Input: part model. Units: mm. Frame: model coordinates. A direction names the side the tool comes from. Round coordinates to 2 decimals unless told otherwise and drop trailing zeros. Order: outer loops, then holes, each group sorted by start corner. A loop starts at its lowest first (then second) coordinate and runs counter-clockwise, first axis right, second up. Notation, with made-up numbers: (2, 84.5) -> (7, 84.5) arc R21 cw to (7, 106.5) -> close; hole circle Ø3 at (41, -8.5). An arc over 180 degrees is marked (long way). Answer as CSV lines item,"result". Start each with the question number.
1) First-contact query: P1, Ø5, axis at x = 20, z = 6, coming from the -Y side; P2, Ø1, axis at y = -2, z = 2, coming from the +X side; P3, Ø4, axis at x = -40, z = 0, coming from the +Y side. Flat tips, straight axial feed; report the tip coordinate or a pass-through.
2) Section query D-D, the plane x = -19.5. Output: boundary loops of the cut face in (y, z).
3) Line query: L1, parallel to X at y = -2.05, z = 0; L2, parallel to Z at x = -40, y = -1.7; L3, parallel to X at y = -2.75, z = -0.25. Output: solid intervals per line, ascending.
4) Section query C-C, the plane x = -5.5. Output: boundary loops of the cut face in (y, z), and give its area (3 significant figures).
5) Access query for faces 5 (the face through (-1, 0, 0)), 6 (the face through (-38.099, -1.268, -9.818)), 7 (the face through (38, -1.3, 9.8)). Directions: +Z, -Z, +X, -X, +Y, -Y. A direction counts if a zero-diameter tool reaches every point of the face in a straight line with its end or side. Return the directions, or none.
6) Section query A-A, the plane y = -0.9. State how many separate pieces and enclosed holes the cut face has, and give its area (3 significant figures).
7) Section query B-B, the plane z = -5.5. Output: boundary loops of the cut face in (x, y), and give its area (3 significant figures).
8) Mould query, pull axis Z, two halves, no side actions, for faces 1 (the face through (-47.15, -1.27, 6.99)), 2 (the face through (42.1, -1.52, -0.09)), 3 (the face through (0.52, -1.232, -2.165)), 4 (the face through (41.3, -3, -2)). Classes: +Z half, -Z half, draft (parallel to the pull), parting line (faces both ways), or undercut.
```python
from build123d import *

# Parameters (mm, degrees)
F0_R     = 6
F1_DEPTH = 2.5
F2_DEPTH = 3
F2_TAPER = 45
F3_D     = 4.2
F4_R     = 9.99999


# Not quite as in the source:
# - a fillet or chamfer is up to 0.001 mm smaller than in the source, because OpenCascade refuses the exact size


with BuildPart() as f1:
    # F0 (on Front) → F1 (new body)
    with BuildSketch(Plane.XZ):
        with BuildLine():
            Line((-50, 16.2119245403), (-50, -10))
            Line((-50, -10), (50, -10))
            Line((50, -10), (50, 16.2119245403))
            ThreePointArc((50, 16.2119245403), (0, 2.1631295345), (-50, 16.2119245403))
        make_face()
        with Locations((-40, 0)):
            Circle(F0_R, mode=Mode.SUBTRACT)
        with Locations((40, 0)):
            Circle(F0_R, mode=Mode.SUBTRACT)
        with Locations((-40, 0)):
            Circle(F0_R)
        with Locations((40, 0)):
            Circle(F0_R)
    extrude(amount=F1_DEPTH)

    # F0 (on Front) → F2 (join)
    with BuildSketch(Plane.XZ):
        with Locations((40, 0)):
            Circle(F0_R)
        with Locations((-40, 0)):
            Circle(F0_R)
    extrude(amount=F2_DEPTH, taper=F2_TAPER)

    # F3 (through all)
    with Locations(Plane(origin=(0, 0, 0), x_dir=(1, 0, 0), z_dir=(0, 1, 0))):
        with Locations((40, 0), (-40, 0)):
            Hole(F3_D / 2)

    # F4 (radius 10 in the source; OpenCascade refuses exactly that, so slightly less here)
    f4_edges = [f1.edges().sort_by_distance(p)[0] for p in [
        (-50, -1.25, 16.211925),
        (50, -1.25, 16.211925),
        (50, -1.25, -10),
        (-50, -1.25, -10),
    ]]
    fillet(f4_edges, radius=F4_R)


with BuildPart() as f5_1:
    # F5: instance of F1
    add(f1.part.mirror(Plane.XY))


with BuildPart() as f1_1:
    add(f1.part)

    # F6: intersect F5_1
    add(f5_1.part, mode=Mode.INTERSECT)


solid = f1_1.part
```
Findings:
1,P1,"stops at y = -2.5"
1,P2,"stops at x = 49.89"
1,P3,"passes through"
2,outline,"(-2.5, -4.16) -> (0, -4.16) -> (0, 4.16) -> (-2.5, 4.16) -> close"
3,L1,"x = -50 to -42.1, -37.9 to 37.9, 42.1 to 50"
3,L2,"z = -10 to -2.1, 2.1 to 10"
3,L3,"x = -43.24 to -42.09, -37.91 to -36.76, 36.76 to 37.91, 42.09 to 43.24"
4,outline,"(-2.5, -2.32) -> (0, -2.32) -> (0, 2.32) -> (-2.5, 2.32) -> close"
4,area,"11.6 mm^2"
5,face 5,"+Z, -Z, +X, -X, +Y"
5,face 6,"-Z, +Y, -Y"
5,face 7,"+Z, +Y, -Y"
6,separate pieces,"1"
6,enclosed holes,"2"
6,area,"1,080 mm^2"
7,outline,"(-48.35, -2.5) -> (-25.09, -2.5) -> (-25.09, 0) -> (-48.35, 0) -> close; (25.09, -2.5) -> (48.35, -2.5) -> (48.35, 0) -> (25.09, 0) -> close"
7,area,"116 mm^2"
8,face 1,"+Z half"
8,face 2,"undercut"
8,face 3,"-Z half"
8,face 4,"draft"
